from build123d import *

# Parameters (mm, degrees)
SKETCH1_R           = 9
BOSS_EXTRUDE1_DEPTH = 32.5
SKETCH2_R           = 7
SKETCH2_R_2         = 4
CUT_EXTRUDE1_DEPTH  = 1
FILLET1_R           = 0.2


with BuildPart() as part:
    # Sketch1 → Boss-Extrude1 (new, symmetric)
    with BuildSketch(Plane.XY):
        Circle(SKETCH1_R)
    extrude(amount=BOSS_EXTRUDE1_DEPTH, both=True)

    # Sketch2 → Cut-Extrude1 (cut)
    with BuildSketch(Plane.XY.offset(32.5)):
        Circle(SKETCH2_R)
        Circle(SKETCH2_R_2, mode=Mode.SUBTRACT)
    extrude(amount=-CUT_EXTRUDE1_DEPTH, mode=Mode.SUBTRACT)

    # Fillet1
    fillet1_edges = [part.edges().sort_by_distance(p)[0] for p in [
        (-4, 0, 32.5),
        (-9, 0, -32.5),
        (-9, 0, 32.5),
    ]]
    fillet(fillet1_edges, radius=FILLET1_R)


solid = part.part
Source: CAD feature listing. Evaluate the final solid. Frame: model axes, mm. A direction names the side the tool comes from. Coordinates: 2 decimals unless noted, no trailing zeros. Loops run counter-clockwise (first coordinate to the right, second up) from the corner with the lowest first, then second, coordinate; pieces in that order, holes last. Notation, with made-up numbers: M 69.5,87.25 L 112.5,87.25 A21 ccw 112.5,94.25 Z; hole C 14.25,-35.75 d5. An arc over 180 degrees is marked long. Answer in a Markdown table with one row per item.
Q1. Section A-A on z = -23.5. Return the cut outline in (x, y).
Answers below:
| item | result |
|---|---|
| outline | C 0,0 d18 |
Q2. Ray query, probe 1 along Y at (x, z) = (0, 32.05); probe 2 along Y at (x, z) = (0, -19); probe 3 along Z at (x, y) = (-5, -3.5). Return the intervals inside material, ascending. Write a range as from..to.
Answers below:
| item | result |
|---|---|
| probe 1 | y = -9..-7, -4..4, 7..9 |
| probe 2 | y = -9..9 |
| probe 3 | z = -32.5..31.5 |
Q3. First-contact query: pin 1 (2 mm diameter, centred on y = -5, z = -10, fed in from -X); pin 2 (6 mm diameter, centred on x = 6, z = 10, fed in from +Y); pin 3 (1.5 mm diameter, centred on x = 1.5, z = -6.5, fed in from +Y). Flat tips, straight axial feed; report the tip coordinate or a pass-through.
Answers below:
| item | result |
|---|---|
| pin 1 | stops at x = -8.06 |
| pin 2 | stops at y = 8.49 |
| pin 3 | stops at y = 8.97 |
Q4. Draft query along Y for faces 3 (the cylindrical face through (-1.172, 8.923, 0.452)), 4 (the flat face through (-6, -4, 32.5)), 5 (the cylindrical face through (6.466, -2.681, 32.007)). Return one class per face: pulls with the +Y half, pulls with the -Y half, needs draft (parallel to the pull), parting line crosses it, or undercut.
Answers below:
| item | result |
|---|---|
| face 3 | parting line crosses it |
| face 4 | needs draft |
| face 5 | undercut |
Q5. Set-up query: faces 1 (the flat face through (0, 0, -32.5)), 2 (the cylindrical face through (-0.867, -3.905, 31.906)). Return all of +Z, -Z, +X, -X, +Y, -Y with unobstructed straight access to the full face (end or side cutting, diameter ignored); none if empty.
Answers below:
| item | result |
|---|---|
| face 1 | -Z, +X, -X, +Y, -Y |
| face 2 | +Z |
